Autodesk Inventor part; units mm, degrees
ref_plane "YZ Plane" through (0, 0, 0) normal (1, 0, 0) x (0, 1, 0)
ref_plane "XZ Plane" through (0, 0, 0) normal (0, 1, 0) x (-1, 0, 0)
ref_plane "XY Plane" through (0, 0, 0) normal (0, 0, 1) x (1, 0, 0)
sketch "Sketch1" plane through (0, 0, 0) normal (0, 0, 1) x (1, 0, 0)
  circle A0 centre (0, 0) radius 101.6
  circle A1 centre (0, 0) radius 127
  dimension "d0" = 203.2
  dimension "d1" = 25.4
extrude "Extrusion1" add sketch "Sketch1" along normal mid plane 101.6
sketch "Sketch2" plane through (0, 0, 50.8) normal (0, 0, 1) x (1, 0, 0)
  circle A0 centre (0, 0) radius 127
  line L0 (-16.5768, 125.9135) -> (-9.1361, 107.95)
  line L1 (-9.1361, 107.95) -> (9.1361, 107.95)
  line L2 (9.1361, 107.95) -> (16.5768, 125.9135)
  line L3 (0, 107.95) -> (0, 128.4311) construction
  line L4 (-16.5768, 125.9135) -> (0, 0) construction
  line L5 (0, 0) -> (16.5768, 125.9135) construction
  arc A1 (16.5768, 125.9135) -> (-16.5768, 125.9135) centre (0, 0) ccw
  dimension "d4" = 19.05
  dimension "d5" = 45
  dimension "d6" = 15
extrude "Extrusion2" cut sketch "Sketch2" against normal through all contours L2 L1 L0 A0 picked at (-1.8466, 114.2597)
pattern_circular "Circular Pattern1" count 20 over 360 about axis through (0, 0, 0) along (0, 0, 1) of "Extrusion2"
properties part number "NASA-20-TRD-01" material "PET Plastic"
The listing builds one solid part. Answer for the finished solid, in the listing's coordinates (mm). A direction names the side the tool comes from. Coordinates: 2 decimals unless noted, no trailing zeros. Loops run counter-clockwise (first coordinate to the right, second up) from the corner with the lowest first, then second, coordinate; pieces in that order, holes last. Notation, with made-up numbers: (10, 26) -> (26, 26) arc R26 cw to (26, 65) -> close; hole circle Ø8 at (23.5, 48). An arc over 180 degrees is marked (long way). Answer in a Markdown table with one row per item. Add a question column.
1. The part is cut by section A-A, the plane x = 0. Write down the section's boundary in (y, z), then the cut area to 3 significant figures.
2. Determine the mould class of faces 5 (the flat face through (48.27, 107.13, 0.71)), 6 (the flat face through (-12.91, 117.06, 0.71)), 7 (the flat face through (102.706, -33.237, 0.711)), 8 (the flat face through (-58.298, 102.024, 0.711)) for opening direction X: +X half, -X half, draft (parallel to the pull), parting line (faces both ways), or undercut.
3. Consider line 1 (Y direction, x = 0, z = 15); line 2 (Y direction, x = 106, z = 6.5); line 3 (Y direction, x = -89.5, z = 3). Determine where each line is inside the solid, lowest interval first. Write a range as [from, to].
4. Flat-ended cylindrical pins translate along their axes: P1, Ø14.5, axis at x = -0.5, z = 21.5, coming from the +Y side; P2, Ø1, axis at y = -79, z = 23.5, coming from the -X side; P3, Ø1, axis at x = 30.5, z = -33, coming from the -Y side. Find the tip coordinate at first contact, or state that the pin passes through.
5. For faces 1 (the flat face through (102.024, 58.298, 0.711)), 2 (the flat face through (115.046, 23.917, 0.711)), 3 (the flat face through (-12.8, -116.8, 0.7)), 4 (the flat face through (-87.26, -63.55, 0.71)), determine the directions among +Z, -Z, +X, -X, +Y, -Y from which every point of the face is accessible in a straight line to the end or side of a thin tool.
Answer below:
| question | item | result |
|---|---|---|
| 1 | outline | (-107.95, -50.8) -> (-101.6, -50.8) -> (-101.6, 50.8) -> (-107.95, 50.8) -> close; (101.6, -50.8) -> (107.95, -50.8) -> (107.95, 50.8) -> (101.6, 50.8) -> close |
| 1 | area | 1,290 mm2 |
| 2 | face 5 | undercut |
| 2 | face 6 | undercut |
| 2 | face 7 | +X half |
| 2 | face 8 | -X half |
| 3 | line 1 | [-107.95, -101.6], [101.6, 107.95] |
| 3 | line 2 | [-59.25, -47.31], [-24.63, 24.63], [47.31, 59.25] |
| 3 | line 3 | [-90.1, -83.14], [-60.47, -48.09], [48.09, 60.47], [83.14, 90.1] |
| 4 | P1 | y = 107.95 |
| 4 | P2 | x = -87.27 |
| 4 | P3 | y = -103.76 |
| 5 | face 1 | +Z, -Z, +Y |
| 5 | face 2 | +Z, -Z, +X |
| 5 | face 3 | +Z, -Z, -Y |
| 5 | face 4 | +Z, -Z |
